Here's how the part is built. I have some questions about the finished solid (model axes, mm). Face numbers are marked on the shaded views. A direction names the side the tool comes from. Round coordinates to 2 decimals unless told otherwise and drop trailing zeros. Loops run counter-clockwise (first coordinate to the right, second up) from the corner with the lowest first, then second, coordinate; pieces in that order, holes last. Notation, with made-up numbers: (-25.5, 65) -> (4.5, 65) arc R12 ccw to (4.5, 69) -> close; hole circle Ø2 at (1, 11.25). An arc over 180 degrees is marked (long way). Use one line per item in the form item = value. Start each with the question number.
Item 1: If we section it at C-C (x = 4.25): Write out the boundary of the cut face in (y, z) (3 decimals), then the cut area to 3 significant figures.
Item 2: If we section it at A-A (z = -2.75): Write out the boundary of the cut face in (x, y), then the cut area to 3 significant figures.
Item 3: I'm going to push flat-ended pins straight in: pin 1 Ø2 at (x, z) = (4, -5) entering from -Y; pin 2 Ø1 at (x, y) = (5, -2) entering from -Z; pin 3 Ø1.5 at (x, y) = (1.5, -3) entering from -Z. Where does each tip first touch, or does it pass through?
Item 4: If we section it at D-D (z = -5.5): Write out the boundary of the cut face in (x, y).
Item 5: Thinking about a two-plate mould opening in Z: for the marked faces 4, 5 and 6, which applies, released by +Z, released by -Z, zero draft, split by the parting line, or undercut?
Item 6: For the marked faces 1, 2 and 3, which set-ups out of +Z, -Z, +X, -X, +Y, -Y let a thin tool reach every point of the face, with its end or its side?
Item 7: If I drill on L1, parallel to Y at x = 8, z = 0 (3 decimals); L2, parallel to X at y = 2.5, z = -6; L3, parallel to Y at x = 9.5, z = 2, over which ranges is the centre line in solid material (lowest first)? Write a range as [from, to].
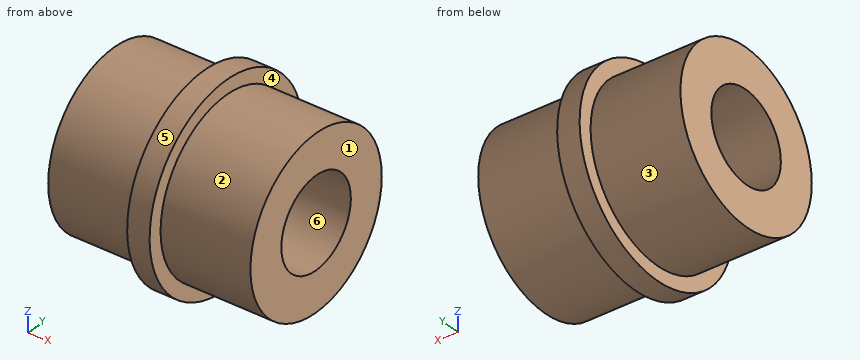
```python
from build123d import *

# Parameters (mm, degrees)
SKETCH1_R           = 5.999999938
BOSS_EXTRUDE1_DEPTH = 6.35
SKETCH2_R           = 6.99999997
BOSS_EXTRUDE2_DEPTH = 1.5875
SKETCH3_R           = 5.999999938
BOSS_EXTRUDE3_DEPTH = 6.35
SKETCH4_R           = 3.175
CUT_EXTRUDE1_DEPTH  = 15.2875


with BuildPart() as part:
    # Sketch1 → Boss-Extrude1 (new body)
    with BuildSketch(Plane(origin=(0, 0, 0), x_dir=(0, 0, -1), z_dir=(1, 0, 0))):
        Circle(SKETCH1_R)
    extrude(amount=BOSS_EXTRUDE1_DEPTH)

    # Sketch2 → Boss-Extrude2 (add)
    with BuildSketch(Plane(origin=(6.35, 0, 0), x_dir=(0, 0, -1), z_dir=(1, 0, 0))):
        Circle(SKETCH2_R)
    extrude(amount=BOSS_EXTRUDE2_DEPTH)

    # Sketch3 → Boss-Extrude3 (add)
    with BuildSketch(Plane(origin=(7.9375, 0, 0), x_dir=(0, 0, -1), z_dir=(1, 0, 0))):
        Circle(SKETCH3_R)
    extrude(amount=BOSS_EXTRUDE3_DEPTH)

    # Sketch4 → Cut-Extrude1 (cut, through all)
    with BuildSketch(Plane(origin=(14.2875, 0, 0), x_dir=(0, 0, -1), z_dir=(1, 0, 0))):
        Circle(SKETCH4_R)
    extrude(amount=-CUT_EXTRUDE1_DEPTH, mode=Mode.SUBTRACT)


solid = part.part
```
Values found:
q1.outline = circle Ø12 at (0, 0); hole circle Ø6.35 at (0, 0)
q1.area = 81.4 mm2
q2.outline = (0, -5.33) -> (6.35, -5.33) -> (6.35, -6.44) -> (7.94, -6.44) -> (7.94, -5.33) -> (14.29, -5.33) -> (14.29, -1.59) -> (0, -1.59) -> close; (0, 1.59) -> (14.29, 1.59) -> (14.29, 5.33) -> (7.94, 5.33) -> (7.94, 6.44) -> (6.35, 6.44) -> (6.35, 5.33) -> (0, 5.33) -> close
q2.area = 111 mm2
q3.pin_1 = -4.47
q3.pin_2 = -5.81
q3.pin_3 = -5.56
q4.outline = (0, -2.4) -> (6.35, -2.4) -> (6.35, -4.33) -> (7.94, -4.33) -> (7.94, -2.4) -> (14.29, -2.4) -> (14.29, 2.4) -> (7.94, 2.4) -> (7.94, 4.33) -> (6.35, 4.33) -> (6.35, 2.4) -> (0, 2.4) -> close
q5.face_4 = zero draft
q5.face_5 = split by the parting line
q5.face_6 = undercut
q6.face_1 = +Z, -Z, +X, +Y, -Y
q6.face_2 = +X
q6.face_3 = -X
q7.L1 = [-6, -3.175], [3.175, 6]
q7.L2 = [6.35, 7.94]
q7.L3 = [-5.66, -2.47], [2.47, 5.66]
